from build123d import *

# Parameters (mm, degrees)
SKETCH1_R                        = 2.5
BOSS_EXTRUDE1_DEPTH              = 12.7
FILLET1_R                        = 3.175
TAP_DRILL_FOR_M10X1_5_TAP1_D     = 8.5
TAP_DRILL_FOR_M10X1_5_TAP1_DEPTH = 20
TAP_DRILL_FOR_M10X1_5_TAP1_TIP   = 2.553657631


with BuildPart() as part:
    # Sketch1 → Boss-Extrude1 (new body)
    with BuildSketch(Plane.XY):
        with BuildLine():
            ThreePointArc((25, 0), (24.117920391, -6.582242475), (21.53392672, -12.7))
            Line((21.53392672, -12.7), (35.496478699, -12.7))
            ThreePointArc((35.496478699, -12.7), (37.145034977, -6.444872111), (37.7, 0))
            ThreePointArc((37.7, 0), (37.145034977, 6.444872111), (35.496478699, 12.7))
            Line((35.496478699, 12.7), (21.53392672, 12.7))
            ThreePointArc((21.53392672, 12.7), (24.117920391, 6.582242475), (25, 0))
        make_face()
        with BuildLine():
            Line((35.496478699, -12.7), (21.53392672, -12.7))
            ThreePointArc((21.53392672, -12.7), (-25, 0), (21.53392672, 12.7))
            Line((21.53392672, 12.7), (35.496478699, 12.7))
            ThreePointArc((35.496478699, 12.7), (-37.7, 0), (35.496478699, -12.7))
        make_face()
        with BuildLine():
            ThreePointArc((37.7, 0), (37.145034977, -6.444872111), (35.496478699, -12.7))
            Line((35.496478699, -12.7), (76.417300015, -12.7))
            Line((76.417300015, -12.7), (76.417300015, 12.7))
            Line((76.417300015, 12.7), (35.496478699, 12.7))
            ThreePointArc((35.496478699, 12.7), (37.145034977, 6.444872111), (37.7, 0))
        make_face()
        with BuildLine():
            Line((-1.017300015, 12.7), (-1.017300015, -12.7))
            Line((-1.017300015, -12.7), (3.552069768, -12.7))
            ThreePointArc((3.552069768, -12.7), (5.775120383, -11.34369837), (7.998170999, -12.7))
            Line((7.998170999, -12.7), (21.53392672, -12.7))
            ThreePointArc((21.53392672, -12.7), (24.117920391, -6.582242475), (25, 0))
            ThreePointArc((25, 0), (24.117920391, 6.582242475), (21.53392672, 12.7))
            Line((21.53392672, 12.7), (7.913288635, 12.7))
            ThreePointArc((7.913288635, 12.7), (5.705346209, 11.372599779), (3.497403783, 12.7))
            Line((3.497403783, 12.7), (-1.017300015, 12.7))
        make_face()
        with Locations((13.872599779, -5.705346209)):
            Circle(SKETCH1_R, mode=Mode.SUBTRACT)
        with Locations((13.84369837, 5.775120383)):
            Circle(SKETCH1_R, mode=Mode.SUBTRACT)
        with BuildLine():
            Line((3.552069768, -12.7), (-1.017300015, -12.7))
            Line((-1.017300015, -12.7), (-1.017300015, 12.7))
            Line((-1.017300015, 12.7), (3.497403783, 12.7))
            ThreePointArc((3.497403783, 12.7), (5.101134353, 16.29848684), (8.205346209, 13.872599779))
            ThreePointArc((8.205346209, 13.872599779), (8.13123327, 13.268387923), (7.913288635, 12.7))
            Line((7.913288635, 12.7), (21.53392672, 12.7))
            ThreePointArc((21.53392672, 12.7), (-25, 0), (21.53392672, -12.7))
            Line((21.53392672, -12.7), (7.998170999, -12.7))
            ThreePointArc((7.998170999, -12.7), (8.204896766, -13.255322019), (8.275120383, -13.84369837))
            ThreePointArc((8.275120383, -13.84369837), (5.186744032, -16.273474753), (3.552069768, -12.7))
        make_face()
        with Locations((-13.84369837, -5.775120383)):
            Circle(SKETCH1_R, mode=Mode.SUBTRACT)
        with Locations((-5.705346209, -13.872599779)):
            Circle(SKETCH1_R, mode=Mode.SUBTRACT)
        with Locations((-13.872599779, 5.705346209)):
            Circle(SKETCH1_R, mode=Mode.SUBTRACT)
        with Locations((-5.775120383, 13.84369837)):
            Circle(SKETCH1_R, mode=Mode.SUBTRACT)
    extrude(amount=BOSS_EXTRUDE1_DEPTH)

    # Fillet1
    fillet1_edges = [part.edges().sort_by_distance(p)[0] for p in [
        (35.496478699, 12.7, 6.35),
        (35.496478699, -12.7, 6.35),
    ]]
    fillet(fillet1_edges, radius=FILLET1_R)

    # Tap Drill for M10x1.5 Tap1
    with Locations(Plane.XY.offset(12.7)):
        with Locations((57.041798974, 0)):
            Hole(TAP_DRILL_FOR_M10X1_5_TAP1_D / 2, depth=TAP_DRILL_FOR_M10X1_5_TAP1_DEPTH)
            with Locations((0, 0, -(TAP_DRILL_FOR_M10X1_5_TAP1_DEPTH + TAP_DRILL_FOR_M10X1_5_TAP1_TIP / 2))):  # 118° drill point
                Cone(0, TAP_DRILL_FOR_M10X1_5_TAP1_D / 2, TAP_DRILL_FOR_M10X1_5_TAP1_TIP, mode=Mode.SUBTRACT)


solid = part.part
Work out the finished part from the listing and answer in its coordinate system (mm). A direction names the side the tool comes from. Round coordinates to 2 decimals unless told otherwise and drop trailing zeros. Loops run counter-clockwise (first coordinate to the right, second up) from the corner with the lowest first, then second, coordinate; pieces in that order, holes last. Notation, with made-up numbers: (63.5, -13.75) - (97.5, -13.75) arc R18 cw to (97.5, 10.25) - close; hole circle Ø7 at (42.5, 26.5). An arc over 180 degrees is marked (long way). Use one line per item in the form item = value. Start each with the question number.
(1) Find section D-D on x = 19.5. Determine the outline of the cut face in (y, z), and give its area (3 significant figures).
(2) Consider line 1 (X direction, y = -7, z = 5.75); line 2 (Y direction, x = 15, z = 11); line 3 (Y direction, x = 57, z = 8.5). Determine where each line is inside the solid, lowest interval first.
(3) Find section A-A on y = 0. Determine the outline of the cut face in (x, z), and give its area (3 significant figures).
(4) Find section C-C on x = -12.5. Determine the outline of the cut face in (y, z).
(5) Determine the mould class of faces 1 (the face through (52.99, 1.28, 6.26)), 2 (the face through (-16.34, -5.67, 6.26)), 3 (the face through (35.889, -13.244, 6.439)), 4 (the face through (6, 1, 0)) for opening direction Y: +Y half, -Y half, draft (parallel to the pull), parting line (faces both ways), or undercut.
(6) Which of the six approach directions +Z, -Z, +X, -X, +Y, -Y give full straight-line access (tool end or side, diameter ignored) to faces 5 (the face through (-37.672, 1.447, 6.261)), 6 (the face through (57, -12.7, 6)), 7 (the face through (57, 12.7, 6))?
(7) Find section B-B on z = 5.75. Give the number of separate pieces and of enclosed holes in the cut face, and give its area (3 significant figures).
(8) Flat-ended cylindrical pins translate along their axes: P1, Ø3, axis at x = 51.5, z = 9, coming from the +Y side; P2, Ø5, axis at y = 14, z = 4, coming from the -X side; P3, Ø1.5, axis at y = -23.5, z = 9, coming from the -X side. Find the tip coordinate at first contact, or state that the pin passes through.
Answer list:
q1.outline = (-32.27, 0) - (32.27, 0) - (32.27, 12.7) - (-32.27, 12.7) - close
q1.area = 820 mm^2
q2.line_1 = -37.04 to -16.02, -11.66 to 11.73, 16.01 to 76.42
q2.line_2 = -34.59 to -7.94, -3.47 to 3.56, 7.99 to 34.59
q2.line_3 = -12.7 to -4.25, 4.25 to 12.7
q3.outline = (-37.7, 0) - (52.79, 0) - (52.79, 12.7) - (-37.7, 12.7) - close; (61.29, 0) - (76.42, 0) - (76.42, 12.7) - (61.29, 12.7) - close
q3.area = 1,340 mm^2
q4.outline = (-35.57, 0) - (-7.88, 0) - (-7.88, 12.7) - (-35.57, 12.7) - close; (-3.67, 0) - (3.62, 0) - (3.62, 12.7) - (-3.67, 12.7) - close; (7.79, 0) - (35.57, 0) - (35.57, 12.7) - (7.79, 12.7) - close
q5.face_1 = undercut
q5.face_2 = undercut
q5.face_3 = -Y half
q5.face_4 = draft
q6.face_5 = +Z, -Z
q6.face_6 = +Z, -Z, +X, -Y
q6.face_7 = +Z, -Z, +X, +Y
q7.separate_pieces = 1
q7.enclosed_holes = 9
q7.area = 5,250 mm^2
q8.P1 = 12.7
q8.P2 = -35.9
q8.P3 = -30.06
